Read the model definition and answer for the solid it produces. Units are mm, in the model's axes. A direction names the side the tool comes from. Round coordinates to 2 decimals unless told otherwise and drop trailing zeros. Loops run counter-clockwise (first coordinate to the right, second up) from the corner with the lowest first, then second, coordinate; pieces in that order, holes last. Notation, with made-up numbers: M 68,-1.75 L 93,-1.75 A19 cw 93,32.25 Z; hole C 22.25,16 d3. An arc over 180 degrees is marked long. Write each question's results on one line, items separated by ' | '.
from build123d import *

# Parameters (mm, degrees)
ESBO_O1_W                 = 46
ESBO_O1_H                 = 46
ESBO_O1_R                 = 19
ESBO_O1_R_2               = 16
ESBO_O1_R_3               = 12.5
RESSALTO_EXTRUS_O1_DEPTH  = 22
ESBO_O1_7_R               = 19
ESBO_O1_7_R_2             = 16
ESBO_O1_7_R_3             = 12.5
RESSALTO_EXTRUS_O4_DEPTH  = 25
RESSALTO_EXTRUS_O5_START  = -3
ESBO_O1_8_R               = 19
ESBO_O1_8_R_2             = 16
ESBO_O1_8_R_3             = 12.5
RESSALTO_EXTRUS_O5_DEPTH  = 3
ESBO_O7_R                 = 8
ESBO_O7_R_2               = 6
RESSALTO_EXTRUS_O8_DEPTH  = 12
RESSALTO_EXTRUS_O9_DEPTH  = 22
RESSALTO_EXTRUS_O10_START = 12
ESBO_O8_R                 = 8
ESBO_O8_R_2               = 6
RESSALTO_EXTRUS_O10_DEPTH = 12
RESSALTO_EXTRUS_O11_START = 22
RESSALTO_EXTRUS_O11_DEPTH = 22


with BuildPart() as part:
    # Esbo_o1 → Ressalto-extrus_o1 (new body)
    # profile 1 of 3: a face of its own
    with BuildSketch(Plane(origin=(0, 0, 0), x_dir=(1, 0, 0), z_dir=(0, 1, 0))):
        Rectangle(ESBO_O1_W, ESBO_O1_H)
        Circle(ESBO_O1_R, mode=Mode.SUBTRACT)
    # profile 2 of 3: a face of its own
    with BuildSketch(Plane(origin=(0, 0, 0), x_dir=(1, 0, 0), z_dir=(0, 1, 0))):
        Circle(ESBO_O1_R)
        Circle(ESBO_O1_R_2, mode=Mode.SUBTRACT)
    # profile 3 of 3: a face of its own
    with BuildSketch(Plane(origin=(0, 0, 0), x_dir=(1, 0, 0), z_dir=(0, 1, 0))):
        Circle(ESBO_O1_R_2)
        with Locations(Location((0, 0, 0), (0, 0, 270))):
            Circle(ESBO_O1_R_3, mode=Mode.SUBTRACT)
    extrude(amount=RESSALTO_EXTRUS_O1_DEPTH)

    # Esbo_o1_7 → Ressalto-extrus_o4 (add)
    # profile 1 of 2: a face of its own
    with BuildSketch(Plane(origin=(0, 0, 0), x_dir=(1, 0, 0), z_dir=(0, 1, 0))):
        with Locations(Location((0, 0, 0), (0, 0, 270))):
            Circle(ESBO_O1_7_R)
        Circle(ESBO_O1_7_R_2, mode=Mode.SUBTRACT)
    # profile 2 of 2: a face of its own
    with BuildSketch(Plane(origin=(0, 0, 0), x_dir=(1, 0, 0), z_dir=(0, 1, 0))):
        Circle(ESBO_O1_7_R_2)
        with Locations(Location((0, 0, 0), (0, 0, 270))):
            Circle(ESBO_O1_7_R_3, mode=Mode.SUBTRACT)
    extrude(amount=RESSALTO_EXTRUS_O4_DEPTH)

    # Esbo_o1_8 → Ressalto-extrus_o5 (add)
    # profile 1 of 2: a face of its own
    with BuildSketch(Plane(origin=(0, 0, 0), x_dir=(1, 0, 0), z_dir=(0, 1, 0)).offset(RESSALTO_EXTRUS_O5_START)):
        with Locations(Location((0, 0, 0), (0, 0, 270))):
            Circle(ESBO_O1_8_R)
        Circle(ESBO_O1_8_R_2, mode=Mode.SUBTRACT)
    # profile 2 of 2: a face of its own
    with BuildSketch(Plane(origin=(0, 0, 0), x_dir=(1, 0, 0), z_dir=(0, 1, 0)).offset(RESSALTO_EXTRUS_O5_START)):
        Circle(ESBO_O1_8_R_2)
        with Locations(Location((0, 0, 0), (0, 0, 270))):
            Circle(ESBO_O1_8_R_3, mode=Mode.SUBTRACT)
    extrude(amount=RESSALTO_EXTRUS_O5_DEPTH)

    # Esbo_o7 → Ressalto-extrus_o8 (add)
    with BuildSketch(Plane.ZY.offset(23)):
        with Locations(Location((0, 11, 0), (0, 0, 180))):
            Circle(ESBO_O7_R)
        with Locations((0, 11)):
            Circle(ESBO_O7_R_2, mode=Mode.SUBTRACT)
    extrude(amount=RESSALTO_EXTRUS_O8_DEPTH)

    # Esbo_o7_3 → Ressalto-extrus_o9 (add)
    with BuildSketch(Plane.ZY.offset(23)):
        with BuildLine():
            ThreePointArc((6, 11), (4.242640687, 15.242640687), (0, 17))
            Line((0, 17), (0, 5))
            ThreePointArc((0, 5), (4.242640687, 6.757359313), (6, 11))
        make_face()
        with BuildLine():
            Line((0, 5), (0, 17))
            ThreePointArc((0, 17), (-6, 11), (0, 5))
        make_face()
    extrude(amount=RESSALTO_EXTRUS_O9_DEPTH)

    # Esbo_o8 → Ressalto-extrus_o10 (add)
    with BuildSketch(Plane(origin=(23, 0, 0), x_dir=(0, 0, -1), z_dir=(1, 0, 0)).offset(RESSALTO_EXTRUS_O10_START)):
        with Locations((0, 11)):
            Circle(ESBO_O8_R)
        with Locations(Location((0, 11, 0), (0, 0, 180))):
            Circle(ESBO_O8_R_2, mode=Mode.SUBTRACT)
    extrude(amount=-RESSALTO_EXTRUS_O10_DEPTH)

    # Esbo_o8_2 → Ressalto-extrus_o11 (add)
    with BuildSketch(Plane(origin=(23, 0, 0), x_dir=(0, 0, -1), z_dir=(1, 0, 0)).offset(RESSALTO_EXTRUS_O11_START)):
        with BuildLine():
            ThreePointArc((6, 11), (4.242640687, 15.242640687), (0, 17))
            Line((0, 17), (0, 5))
            ThreePointArc((0, 5), (4.242640687, 6.757359313), (6, 11))
        make_face()
        with BuildLine():
            Line((0, 5), (0, 17))
            ThreePointArc((0, 17), (-6, 11), (0, 5))
        make_face()
    extrude(amount=-RESSALTO_EXTRUS_O11_DEPTH)


solid = part.part
Item 1: The part is cut by section C-C (y = 20.75). Determine the outline of the cut face in (x, z).
Outcome:
outline: M -23,-23 L 23,-23 L 23,23 L -23,23 Z; hole C 0,0 d25
Item 2: For faces 1 (the face through (-21, 22, 0)), 2 (the face through (35, 17, 2)), 3 (the face through (0, 11, 23)), 4 (the face through (-11.56, -1.52, -15.08)), 5 (the face through (-35, 5, 2)), determine the directions among +Z, -Z, +X, -X, +Y, -Y from which every point of the face is accessible in a straight line to the end or side of a thin tool.
Outcome:
face 1: +Y | face 2: +X | face 3: +Z, +X, -X, +Y, -Y | face 4: -Y | face 5: -X
Item 3: The mould has two halves that part along Z. Classify faces 6 (the face through (-11.56, 23.48, -15.08)), 7 (the face through (23, 18, 5)), 8 (the face through (3.755, 10.804, 11.923)): pulls with the +Z half, pulls with the -Z half, needs draft (parallel to the pull), parting line crosses it, or undercut.
Outcome:
face 6: parting line crosses it | face 7: needs draft | face 8: undercut
Item 4: Flat-ended cylindrical pins translate along their axes: pin 1 (1.5 mm diameter, centred on y = 1, z = -17.5, fed in from -X); pin 2 (6 mm diameter, centred on x = -24.5, z = 7, fed in from +Y); pin 3 (3 mm diameter, centred on y = 1.5, z = 1.5, fed in from +X). Find the tip coordinate at first contact, or state that the pin passes through.
Outcome:
pin 1: stops at x = -23 | pin 2: stops at y = 22 | pin 3: stops at x = 23
Item 5: The part is cut by section D-D (z = 16). Determine the outline of the cut face in (x, y).
Outcome:
outline: M -23,0 L -10.25,0 L -10.25,-3 L 10.25,-3 L 10.25,0 L 23,0 L 23,22 L 10.25,22 L 10.25,25 L -10.25,25 L -10.25,22 L -23,22 Z
Item 6: Straight lines are drawn through the part: line 1 (X direction, y = 10, z = 0); line 2 (Y direction, x = 10, z = -16.5); line 3 (X direction, y = 18.5, z = -3.5). For each, find the intervals that lie inside material, in ascending order.
Outcome:
line 1: x = -45 to -12.5, 12.5 to 45 | line 2: y = 0 to 22 | line 3: x = -23 to -12, 12 to 23
Item 7: The part is cut by section A-A (x = 0). Determine the outline of the cut face in (y, z).
Outcome:
outline: M -3,-19 L 0,-19 L 0,-23 L 22,-23 L 22,-19 L 25,-19 L 25,-12.5 L -3,-12.5 Z; M -3,12.5 L 25,12.5 L 25,19 L 22,19 L 22,23 L 0,23 L 0,19 L -3,19 Z
